```python
from build123d import *

# Parameters (mm, degrees)
SKETCH1_R           = 3.75
BOSS_EXTRUDE1_DEPTH = 4
SKETCH2_R           = 2.3
CUT_EXTRUDE1_DEPTH  = 1
BOSS_EXTRUDE2_START = -1.5
SKETCH3_R           = 0.5
BOSS_EXTRUDE2_DEPTH = 1.5
SKETCH4_R           = 1.25
CUT_EXTRUDE2_DEPTH  = 4.5
CUT_EXTRUDE3_START  = -2.5
SKETCH5_R           = 2.3
CUT_EXTRUDE3_DEPTH  = 2.5


with BuildPart() as part:
    # Sketch1 → Boss-Extrude1 (new body)
    with BuildSketch(Plane(origin=(0, 0, 0), x_dir=(1, 0, 0), z_dir=(0, 1, 0))):
        with Locations(Location((0, 0, 0), (0, 0, 270))):
            Circle(SKETCH1_R)
    extrude(amount=BOSS_EXTRUDE1_DEPTH)

    # Sketch2 → Cut-Extrude1 (cut)
    with BuildSketch(Plane(origin=(0, 4, 0), x_dir=(1, 0, 0), z_dir=(0, 1, 0))):
        with Locations(Location((0, 0, 0), (0, 0, 270))):
            Circle(SKETCH2_R)
    extrude(amount=-CUT_EXTRUDE1_DEPTH, mode=Mode.SUBTRACT)

    # Sketch3 → Boss-Extrude2 (add)
    # profile 1 of 2: a face of its own
    with BuildSketch(Plane(origin=(0, 4, 0), x_dir=(1, 0, 0), z_dir=(0, 1, 0)).offset(BOSS_EXTRUDE2_START)):
        with BuildLine():
            Line((-14.168399438, 1.992897797), (-2.25, 3))
            ThreePointArc((-2.25, 3), (-3.75, 0), (-2.25, -3))
            Line((-2.25, -3), (-14.168399438, -1.992897797))
            ThreePointArc((-14.168399438, -1.992897797), (-16, 0), (-14.168399438, 1.992897797))
        make_face()
        with Locations(Location((-15, 0, 0), (0, 0, 270))):
            Circle(SKETCH3_R, mode=Mode.SUBTRACT)
        with Locations(Location((-13, 0, 0), (0, 0, 270))):
            Circle(SKETCH3_R, mode=Mode.SUBTRACT)
        with Locations(Location((-11, 0, 0), (0, 0, 270))):
            Circle(SKETCH3_R, mode=Mode.SUBTRACT)
        with Locations(Location((-9, 0, 0), (0, 0, 270))):
            Circle(SKETCH3_R, mode=Mode.SUBTRACT)
        with Locations(Location((-7, 0, 0), (0, 0, 270))):
            Circle(SKETCH3_R, mode=Mode.SUBTRACT)
        with Locations(Location((-5, 0, 0), (0, 0, 270))):
            Circle(SKETCH3_R, mode=Mode.SUBTRACT)
    # profile 2 of 2: a face of its own
    with BuildSketch(Plane(origin=(0, 4, 0), x_dir=(1, 0, 0), z_dir=(0, 1, 0)).offset(BOSS_EXTRUDE2_START)):
        with BuildLine():
            Line((14.168399438, -1.992897797), (2.25, -3))
            ThreePointArc((2.25, -3), (3.75, 0), (2.25, 3))
            Line((2.25, 3), (14.168399438, 1.992897797))
            ThreePointArc((14.168399438, 1.992897797), (16, 0), (14.168399438, -1.992897797))
        make_face()
        with Locations(Location((15, 0, 0), (0, 0, 90))):
            Circle(SKETCH3_R, mode=Mode.SUBTRACT)
        with Locations(Location((5, 0, 0), (0, 0, 90))):
            Circle(SKETCH3_R, mode=Mode.SUBTRACT)
        with Locations(Location((7, 0, 0), (0, 0, 90))):
            Circle(SKETCH3_R, mode=Mode.SUBTRACT)
        with Locations(Location((9, 0, 0), (0, 0, 90))):
            Circle(SKETCH3_R, mode=Mode.SUBTRACT)
        with Locations(Location((11, 0, 0), (0, 0, 90))):
            Circle(SKETCH3_R, mode=Mode.SUBTRACT)
        with Locations(Location((13, 0, 0), (0, 0, 90))):
            Circle(SKETCH3_R, mode=Mode.SUBTRACT)
    extrude(amount=BOSS_EXTRUDE2_DEPTH)

    # Sketch4 → Cut-Extrude2 (cut)
    with BuildSketch(Plane(origin=(0, 3, 0), x_dir=(1, 0, 0), z_dir=(0, 1, 0))):
        with Locations(Location((0, 0, 0), (0, 0, 270))):
            Circle(SKETCH4_R)
    extrude(amount=-CUT_EXTRUDE2_DEPTH, mode=Mode.SUBTRACT)

    # Sketch5 → Cut-Extrude3 (cut)
    with BuildSketch(Plane.XZ.offset(CUT_EXTRUDE3_START)):
        with Locations(Location((0, 0, 0), (0, 0, 90))):
            Circle(SKETCH5_R)
    extrude(amount=CUT_EXTRUDE3_DEPTH, mode=Mode.SUBTRACT)


solid = part.part
```
For this review, take the finished solid that the model builds, in its own axes (mm). A direction names the side the tool comes from. Give positions to 0.01 mm unless a question says otherwise; leave off trailing zeros. Write each loop counter-clockwise with the first axis right and the second up, starting at its lowest first coordinate (ties: lowest second). Pieces come first, ordered by that corner, then holes. Notation, with made-up numbers: M -12.5,29.5 L 43.5,29.5 A9 cw 43.5,41.5 Z; hole C -25,-10.5 d10. An arc over 180 degrees is marked long. One line per item, written item: value.
1) For P1, Ø3.5, axis at x = 0, z = 0, coming from the +Y side; P2, Ø3, axis at x = 8, z = -1, coming from the -Y side; P3, Ø1.5, axis at x = -12, y = 3.5, coming from the +Z side, all flat-tipped, find the tip position at first contact; note any pin that passes through.
Results are:
P1: stops at y = 3
P2: stops at y = 2.5
P3: stops at z = 2.24
2) The part is to be moulded in two halves that separate along Z. For faces 1 (the flat face through (8.29, 3.24, 2.49)), 2 (the flat face through (8.126, 3.24, -2.503)), 3 (the cylindrical face through (-13.444, 3.24, 0.231)), 4 (the flat face through (-9, 2.5, 1)), say which applies: +Z half, -Z half, draft (parallel to the pull), parting line (faces both ways), or undercut.
Results are:
face 1: +Z half
face 2: -Z half
face 3: undercut
face 4: draft
3) For faces 5 (the cylindrical face through (-0.691, 1.268, 2.194)), 6 (the flat face through (-8.126, 3.24, 2.503)), 7 (the cylindrical face through (0.691, 3.507, 2.194)), list the 3-axis set-ups (+Z, -Z, +X, -X, +Y, -Y) from which the entire face can be reached by the end or side of a thin tool; tool diameter is ignored.
Results are:
face 5: -Y
face 6: +Z, -X, +Y, -Y
face 7: +Y
4) Take a section at A-A, the plane x = 0. Write out the cut boundary in (y, z), then the cut area to 4 significant figures.
Results are:
outline: M 0,-3.75 L 4,-3.75 L 4,-2.3 L 3,-2.3 L 3,-1.25 L 2.5,-1.25 L 2.5,-2.3 L 0,-2.3 Z; M 0,2.3 L 2.5,2.3 L 2.5,1.25 L 3,1.25 L 3,2.3 L 4,2.3 L 4,3.75 L 0,3.75 Z
area: 12.65 mm²
5) Take a section at C-C, the plane y = 0.45. Write out the cut boundary in (x, z), then the cut area to 3 significant figures.
Results are:
outline: C 0,0 d7.5; hole C 0,0 d4.6
area: 27.6 mm²
6) For line 1 (X direction, y = 0.7, z = 0); line 2 (Y direction, x = -4, z = -1.5); line 3 (Z direction, x = 0.5, y = 0.2) (3 decimals), list the stretches that pass through material, from the lowest coordinate up. Write a range as from..to.
Results are:
line 1: x = -3.75..-2.3, 2.3..3.75
line 2: y = 2.5..4
line 3: z = -3.717..-2.245, 2.245..3.717
7) Take a section at B-B, the plane y = 3.45. Count the separate pieces of the cut face and the enclosed holes in it, then the cut area to 3 significant figures.
Results are:
separate pieces: 1
enclosed holes: 13
area: 136 mm²
